from build123d import *

# Parameters (mm, degrees)
DODANIE_WYCI_GNI_CIE1_DEPTH = 5


with BuildPart() as part:
    # Szkic1 → Dodanie-wyciągnięcie1 (new body)
    with BuildSketch(Plane.XY):
        with BuildLine():
            Line((18, 0), (18, -12.05974013))
            ThreePointArc((18, -12.05974013), (18.568288959, -13.431711041), (19.94025987, -14))
            Line((19.94025987, -14), (22.05974013, -14))
            ThreePointArc((22.05974013, -14), (23.431711041, -13.431711041), (24, -12.05974013))
            Line((24, -12.05974013), (24, 9))
            ThreePointArc((24, 9), (22.535533906, 12.535533906), (19, 14))
            Line((19, 14), (4, 14))
            ThreePointArc((4, 14), (2.585786438, 14.585786438), (2, 16))
            Line((2, 16), (2, 19))
            ThreePointArc((2, 19), (0, 21), (-2, 19))
            Line((-2, 19), (-2, 16))
            ThreePointArc((-2, 16), (-2.585786438, 14.585786438), (-4, 14))
            Line((-4, 14), (-19, 14))
            ThreePointArc((-19, 14), (-22.535533906, 12.535533906), (-24, 9))
            Line((-24, 9), (-24, -12.05974013))
            ThreePointArc((-24, -12.05974013), (-23.431711041, -13.431711041), (-22.05974013, -14))
            Line((-22.05974013, -14), (-19.94025987, -14))
            ThreePointArc((-19.94025987, -14), (-18.568288959, -13.431711041), (-18, -12.05974013))
            Line((-18, -12.05974013), (-18, 0))
            ThreePointArc((-18, 0), (-15, 3), (-12, 0))
            Line((-12, 0), (-12, -12.05974013))
            ThreePointArc((-12, -12.05974013), (-11.431711041, -13.431711041), (-10.05974013, -14))
            Line((-10.05974013, -14), (10.05974013, -14))
            ThreePointArc((10.05974013, -14), (11.431711041, -13.431711041), (12, -12.05974013))
            Line((12, -12.05974013), (12, 0))
            ThreePointArc((12, 0), (15, 3), (18, 0))
        make_face()
    extrude(amount=DODANIE_WYCI_GNI_CIE1_DEPTH)


solid = part.part
Geometry check sheet. Reference: the model listing, model coordinates, mm. A direction names the side the tool comes from. Coordinates: 2 decimals unless noted, no trailing zeros. Order: outer loops, then holes, each group sorted by start corner. A loop starts at its lowest first (then second) coordinate and runs counter-clockwise, first axis right, second up. Notation, with made-up numbers: (46, -16.5) -> (79, -16.5) arc R21 ccw to (79, -4.5) -> close; hole circle Ø6 at (68.5, 51). An arc over 180 degrees is marked (long way). Use a Markdown table: item, result. Add a question column.
1. Cross-section at A-A (y = -11.5). Enter the section's corners in (x, z).
2. Mould release check, pull along X, two halves, no side actions. Record for faces 1 (the face through (0, 21, 2)), 2 (the face through (-11, 14, 2)), 3 (the face through (-18.583, -13.447, 2.465)), 4 (the face through (15, 3, 2)): pulls with the +X half, pulls with the -X half, needs draft (parallel to the pull), parting line crosses it, or undercut.
3. Set-up check for faces 5 (the face through (18, -6, 2)), 6 (the face through (2, 17, 2)), 7 (the face through (21, -14, 2)): record each of +Z, -Z, +X, -X, +Y, -Y from which the full face is reachable in a straight line by a thin tool's end or side.
4. Cross-section at D-D (y = 18.5). Enter the section's corners in (x, z), and give its area (3 significant figures).
5. Go/stop test with flat-tipped pins: pin 1 Ø2.5 at (x, z) = (-10.5, 3.5) entering from +Y; pin 2 Ø5 at (x, y) = (-4.5, 0.5) entering from -Z; pin 3 Ø1 at (y, z) = (10, 3) entering from +X; pin 4 Ø0.9 at (y, z) = (18, 3) entering from +X. Record where each tip stops, or that it passes through.
6. Cross-section at C-C (x = 5.5). Enter the section's corners in (y, z).
7. Cross-section at B-B (z = 2.05). Enter the section's corners in (x, y).
8. Material ranges on L1, parallel to X at y = -3, z = 0.8; L2, parallel to X at y = 16, z = 2.1; L3, parallel to Y at x = -9.5, z = 0.45, recorded low to high.
Filled sheet:
| question | item | result |
|---|---|---|
| 1 | outline | (-24, 0) -> (-18, 0) -> (-18, 5) -> (-24, 5) -> close; (-12, 0) -> (12, 0) -> (12, 5) -> (-12, 5) -> close; (18, 0) -> (24, 0) -> (24, 5) -> (18, 5) -> close |
| 2 | face 1 | parting line crosses it |
| 2 | face 2 | needs draft |
| 2 | face 3 | undercut |
| 2 | face 4 | undercut |
| 3 | face 5 | +Z, -Z, -Y |
| 3 | face 6 | +Z, -Z, +X, +Y |
| 3 | face 7 | +Z, -Z, +X, -X, -Y |
| 4 | outline | (-2, 0) -> (2, 0) -> (2, 5) -> (-2, 5) -> close |
| 4 | area | 20.0 mm2 |
| 5 | pin 1 | y = 14 |
| 5 | pin 2 | z = 0 |
| 5 | pin 3 | x = 23.97 |
| 5 | pin 4 | x = 2 |
| 6 | outline | (-14, 0) -> (14, 0) -> (14, 5) -> (-14, 5) -> close |
| 7 | outline | (-24, -12.06) arc R1.94 ccw to (-22.06, -14) -> (-19.94, -14) arc R1.94 ccw to (-18, -12.06) -> (-18, 0) arc R3 cw to (-12, 0) -> (-12, -12.06) arc R1.94 ccw to (-10.06, -14) -> (10.06, -14) arc R1.94 ccw to (12, -12.06) -> (12, 0) arc R3 cw to (18, 0) -> (18, -12.06) arc R1.94 ccw to (19.94, -14) -> (22.06, -14) arc R1.94 ccw to (24, -12.06) -> (24, 9) arc R5 ccw to (19, 14) -> (4, 14) arc R2 cw to (2, 16) -> (2, 19) arc R2 ccw to (-2, 19) -> (-2, 16) arc R2 cw to (-4, 14) -> (-19, 14) arc R5 ccw to (-24, 9) -> close |
| 8 | L1 | -24 to -18, -12 to 12, 18 to 24 |
| 8 | L2 | -2 to 2 |
| 8 | L3 | -14 to 14 |
